The figure shows three views and two pictorial views of one solid part (mm, origin at its lowest corner). Answer the questions. A direction names the side the tool comes from. Coordinates: 2 decimals unless noted, no trailing zeros. Order: outer loops, then holes, each group sorted by start corner. A loop starts at its lowest first (then second) coordinate and runs counter-clockwise, first axis right, second up. Notation, with made-up numbers: (49, -8) -> (78, -8) arc R28 ccw to (78, 21) -> close; hole circle Ø7 at (68, 30). An arc over 180 degrees is marked (long way). Return JSON: item names as keys, results as strings. Group by question number.
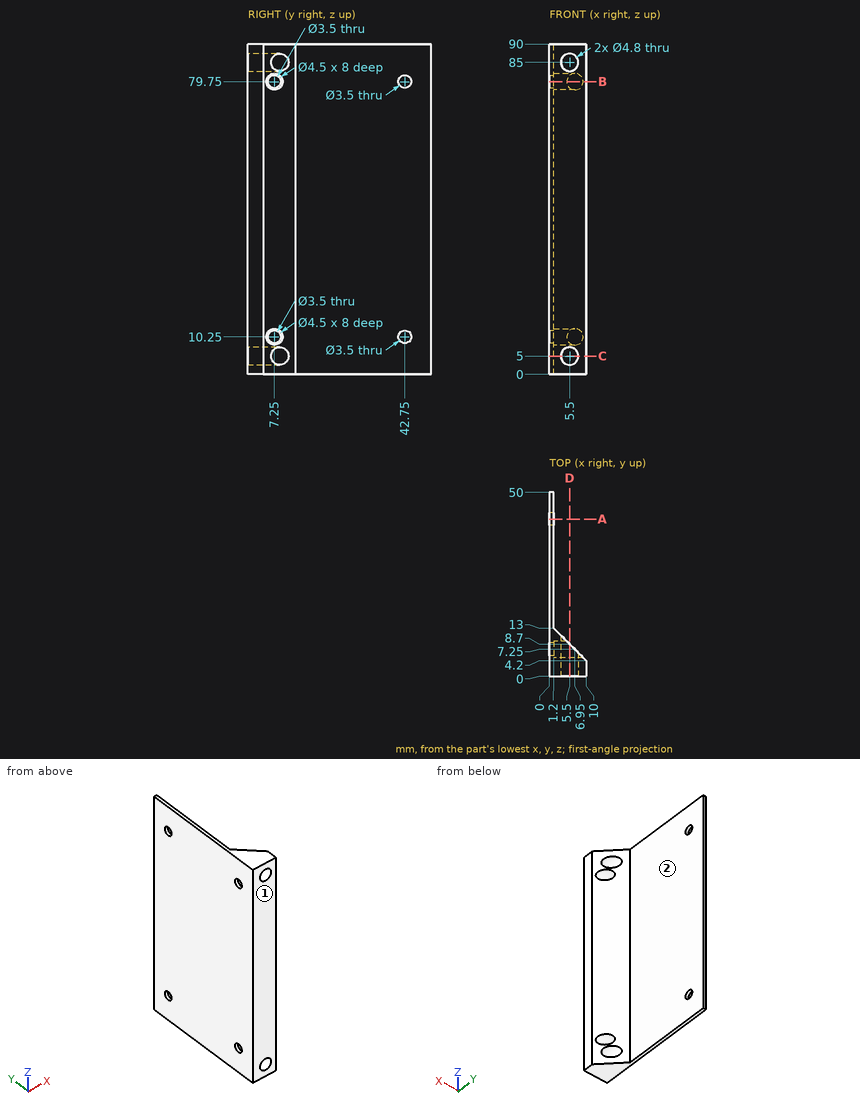
1. Given pin 1 (4.5 mm diameter, centred on x = 5.5, z = 85, fed in from -Y); pin 2 (2 mm diameter, centred on y = 6, z = 25.5, fed in from +X); pin 3 (2 mm diameter, centred on x = 7.5, z = 21.5, fed in from +Y); pin 4 (3 mm diameter, centred on y = 43, z = 54, fed in from +X), each flat-ended and moving along its own axis, determine where each tip first touches the part or whether it passes through.
2. Which of the six approach directions +Z, -Z, +X, -X, +Y, -Y give full straight-line access (tool end or side, diameter ignored) to the marked faces 1 and 2?
3. Straight lines are drawn through the part: L1, parallel to Z at x = 5.5, y = 7.25; L2, parallel to Z at x = 1.25, y = 5.5; L3, parallel to Z at x = 6.25, y = 7.25. For each, find the intervals that lie inside material, in ascending order.
4. Find section A-A on y = 42.75. Determine the outline of the cut face in (x, z).
5. Find section B-B on z = 79.75. Determine the outline of the cut face in (x, y).
6. Find section D-D on x = 5.5. Determine the outline of the cut face in (y, z), and give its area (3 significant figures).
7. Find section C-C on z = 5. Determine the outline of the cut face in (x, y), and give its area (3 significant figures).
Result:
{
 "1": {"pin 1": "through", "pin 2": "x = 9.2", "pin 3": "y = 7.7", "pin 4": "x = 1.2"},
 "2": {"face 1": "+Z, -Z, +X, -X, -Y", "face 2": "+Z, -Z, +X, +Y"},
 "3": {"L1": "0 to 2.6, 7.4 to 8, 12.5 to 77.5, 82 to 82.6, 87.4 to 90", "L2": "0 to 8.84, 11.66 to 78.34, 81.16 to 90", "L3": "0 to 2.72, 7.28 to 8, 12.5 to 77.5, 82 to 82.72, 87.28 to 90"},
 "4": {"outline": "(0, 0) -> (1.2, 0) -> (1.2, 8.5) -> (0, 8.5) -> close; (0, 12) -> (1.2, 12) -> (1.2, 78) -> (0, 78) -> close; (0, 81.5) -> (1.2, 81.5) -> (1.2, 90) -> (0, 90) -> close"},
 "5": {"outline": "(0, 0) -> (10, 0) -> (10, 4.2) -> (9.2, 5) -> (1.2, 5) -> (1.2, 5.5) -> (0, 5.5) -> close; (0, 9) -> (1.2, 9) -> (1.2, 9.5) -> (4.7, 9.5) -> (1.2, 13) -> (1.2, 41) -> (0, 41) -> close; (0, 44.5) -> (1.2, 44.5) -> (1.2, 50) -> (0, 50) -> close"},
 "6": {"outline": "(0, 0) -> (8.7, 0) -> (8.7, 2.6) -> (0, 2.6) -> close; (0, 7.4) -> (8.7, 7.4) -> (8.7, 8.53) arc R2.25 cw (long way) to (8.7, 11.97) -> (8.7, 78.03) arc R2.25 cw (long way) to (8.7, 81.47) -> (8.7, 82.6) -> (0, 82.6) -> close; (0, 87.4) -> (8.7, 87.4) -> (8.7, 90) -> (0, 90) -> close", "area": "671 mm^2"},
 "7": {"outline": "(0, 0) -> (3.1, 0) -> (3.1, 11.1) -> (1.2, 13) -> (1.2, 50) -> (0, 50) -> close; (7.9, 0) -> (10, 0) -> (10, 4.2) -> (7.9, 6.3) -> close", "area": "93.9 mm^2"}
}
